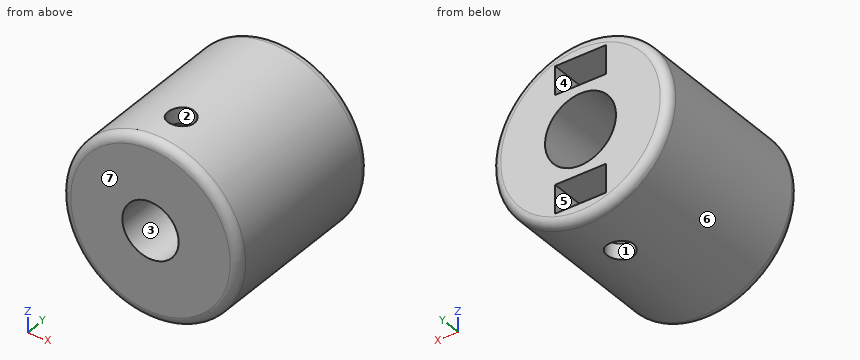
```python
from build123d import *

# Parameters (mm, degrees)
SKETCH1_R           = 10
SKETCH1_R_2         = 3.175
BOSS_EXTRUDE1_DEPTH = 20
SKETCH2_W           = 5.7
SKETCH2_H           = 3.2
CUT_EXTRUDE1_DEPTH  = 17
CUT_EXTRUDE2_DEPTH  = 3.3
SKETCH4_R           = 4
CUT_EXTRUDE3_DEPTH  = 9.3
SKETCH5_W           = 5.7
SKETCH5_H           = 3.2
CUT_EXTRUDE5_DEPTH  = 7.8
CUT_EXTRUDE6_DEPTH  = 3.2
FILLET1_R           = 1
SKETCH7_R           = 1.5
CUT_EXTRUDE7_DEPTH  = 10.2
SKETCH8_R           = 1.5
CUT_EXTRUDE8_DEPTH  = 7.2


with BuildPart() as part:
    # Sketch1 → Boss-Extrude1 (new body)
    with BuildSketch(Plane(origin=(0, 0, 0), x_dir=(1, 0, 0), z_dir=(0, 1, 0))):
        with Locations(Location((0, 0, 0), (0, 0, 270))):
            Circle(SKETCH1_R)
        with Locations(Location((0, 0, 0), (0, 0, 270))):
            Circle(SKETCH1_R_2, mode=Mode.SUBTRACT)
    extrude(amount=BOSS_EXTRUDE1_DEPTH)

    # Sketch2 → Cut-Extrude1 (cut)
    with BuildSketch(Plane(origin=(0, 20, 0), x_dir=(1, 0, 0), z_dir=(0, 1, 0))):
        with Locations((0, -6.5875)):
            Rectangle(SKETCH2_W, SKETCH2_H)
    extrude(amount=-CUT_EXTRUDE1_DEPTH, mode=Mode.SUBTRACT)

    # Sketch3 → Cut-Extrude2 (cut)
    with BuildSketch(Plane.XY.offset(4.9875)):
        Polygon((-2.85, 3), (0, 1.451324557), (2.85, 3), align=None)
    extrude(amount=CUT_EXTRUDE2_DEPTH, mode=Mode.SUBTRACT)

    # Sketch4 → Cut-Extrude3 (cut)
    with BuildSketch(Plane(origin=(0, 20, 0), x_dir=(1, 0, 0), z_dir=(0, 1, 0))):
        with Locations(Location((0, 0, 0), (0, 0, 270))):
            Circle(SKETCH4_R)
    extrude(amount=-CUT_EXTRUDE3_DEPTH, mode=Mode.SUBTRACT)

    # Sketch5 → Cut-Extrude5 (cut)
    with BuildSketch(Plane(origin=(0, 20, 0), x_dir=(1, 0, 0), z_dir=(0, 1, 0))):
        with Locations((0, 6.5875)):
            Rectangle(SKETCH5_W, SKETCH5_H)
    extrude(amount=-CUT_EXTRUDE5_DEPTH, mode=Mode.SUBTRACT)

    # Sketch6 → Cut-Extrude6 (cut)
    with BuildSketch(Plane(origin=(0, 0, -4.9875), x_dir=(-1, 0, 0), z_dir=(0, 0, -1))):
        Polygon((-2.85, 12.2), (0, 10.7), (2.85, 12.2), align=None)
    extrude(amount=CUT_EXTRUDE6_DEPTH, mode=Mode.SUBTRACT)

    # Fillet1
    fillet1_edges = [part.edges().sort_by_distance(p)[0] for p in [
        (0, 0, -10),
        (0, 20, -10),
    ]]
    fillet(fillet1_edges, radius=FILLET1_R)

    # Sketch7 → Cut-Extrude7 (cut)
    with BuildSketch(Plane(origin=(0, 0, -4.9875), x_dir=(-1, 0, 0), z_dir=(0, 0, -1))):
        with Locations(Location((0, 13.836807089, 0), (0, 0, 90))):
            Circle(SKETCH7_R)
    extrude(amount=CUT_EXTRUDE7_DEPTH, mode=Mode.SUBTRACT)

    # Sketch8 → Cut-Extrude8 (cut)
    with BuildSketch(Plane.XY.offset(4.9875)):
        with Locations(Location((0, 4.748303772, 0), (0, 0, 180))):
            Circle(SKETCH8_R)
    extrude(amount=CUT_EXTRUDE8_DEPTH, mode=Mode.SUBTRACT)


solid = part.part
```
For this review, take the finished solid that the model builds, in its own axes (mm). Face numbers are marked on the shaded views. A direction names the side the tool comes from. Round coordinates to 2 decimals unless told otherwise and drop trailing zeros. Write each loop counter-clockwise with the first axis right and the second up, starting at its lowest first coordinate (ties: lowest second). Pieces come first, ordered by that corner, then holes. Notation, with made-up numbers: (19, 13.5) -> (58, 13.5) arc R21 cw to (58, 47.5) -> close; hole circle Ø1 at (32.5, -34). An arc over 180 degrees is marked (long way). Use one line per item in the form item = value.
1) Mouldability with a two-part tool opening along Z and no side actions: class the marked faces 5, 6 and 7 as +Z half, -Z half, draft (parallel to the pull), parting line (faces both ways), or undercut.
Found:
face_5 = undercut
face_6 = parting line
face_7 = draft
2) Tool access review of the marked faces 1, 2, 3 and 4: name each direction out of +Z, -Z, +X, -X, +Y, -Y from which nothing blocks a thin tool from reaching the whole face with its end or side.
Found:
face_1 = -Z
face_2 = +Z
face_3 = +Y, -Y
face_4 = +Y
3) Clearance check with flat-ended pins moving along their axes: pin 1 (2.5 mm diameter, centred on y = 12.5, z = 7, fed in from -X); pin 2 (1 mm diameter, centred on y = 9.5, z = 7.5, fed in from +X); pin 3 (8 mm diameter, centred on y = 10.5, z = -4.5, fed in from -X). State where each tip first meets the part, or that it passes through.
Found:
pin_1 = -8.18
pin_2 = 7.14
pin_3 = -9.99
4) To check wall thickness, follow L1, parallel to Z at x = 0, y = 6.5 (1 decimal); L2, parallel to X at y = 6, z = 0 (3 decimals); L3, parallel to Z at x = 2.5, y = 5. State the ranges of each line that lie inside material, in increasing order. Write a range as from..to.
Found:
L1 = -10..-3.2, 3.2..5, 8.2..10
L2 = -10..-3.175, 3.175..10
L3 = -9.68..-1.96, 1.96..4.99, 8.19..9.68
5) Take a section at B-B, the plane y = 11. Write out the cut boundary in (x, z).
Found:
outline = circle Ø20 at (0, 0); hole circle Ø8 at (0, 0); hole (-2.85, 4.99) -> (2.85, 4.99) -> (2.85, 8.19) -> (-2.85, 8.19) -> close; hole (-0.57, -8.19) -> (0.57, -8.19) -> (0.57, -4.99) -> (-0.57, -4.99) -> close
6) Take a section at C-C, the plane y = 1.75. Count the separate pieces of the cut face and the enclosed holes in it, and give its area (3 significant figures).
Found:
separate_pieces = 1
enclosed_holes = 2
area = 279 mm2
7) Take a section at A-A, the plane z = 0. Write out the cut boundary in (x, y) (3 decimals), and give its area (3 significant figures).
Found:
outline = (-10, 1) arc R1 ccw to (-9, 0) -> (-3.175, 0) -> (-3.175, 10.7) -> (-4, 10.7) -> (-4, 20) -> (-9, 20) arc R1 ccw to (-10, 19) -> close; (3.175, 0) -> (9, 0) arc R1 ccw to (10, 1) -> (10, 19) arc R1 ccw to (9, 20) -> (4, 20) -> (4, 10.7) -> (3.175, 10.7) -> close
area = 257 mm2
